Design review of the part built by this model. Coordinates are the model's own, in mm. A direction names the side the tool comes from. Coordinates: 2 decimals unless noted, no trailing zeros. Loops run counter-clockwise (first coordinate to the right, second up) from the corner with the lowest first, then second, coordinate; pieces in that order, holes last. Notation, with made-up numbers: M 43.25,33.25 L 91.25,33.25 A31 ccw 91.25,64.25 Z; hole C 66,45.25 d2. An arc over 180 degrees is marked long. One line per item, written item: value.
```python
from build123d import *

# Parameters (mm, degrees)
SKETCH1_R           = 1
BOSS_EXTRUDE1_DEPTH = 3
SKETCH2_R           = 5
CUT_EXTRUDE1_DEPTH  = 10
SKETCH4_W           = 3
SKETCH4_H           = 20
BOSS_EXTRUDE3_DEPTH = 3


with BuildPart() as part:
    # Sketch1 → Boss-Extrude1 (new body)
    with BuildSketch(Plane.XY):
        with BuildLine():
            Line((-16.174411119, 11.763860972), (32, 78))
            Line((32, 78), (32, 48))
            Line((32, 48), (19.455095298, -4.636730199))
            ThreePointArc((19.455095298, -4.636730199), (-8.362748941, -18.167675419), (-16.174411119, 11.763860972))
        make_face()
        with Locations((0, 16.5)):
            Circle(SKETCH1_R, mode=Mode.SUBTRACT)
        with Locations((-16.5, 0)):
            Circle(SKETCH1_R, mode=Mode.SUBTRACT)
        with Locations((0, -16.5)):
            Circle(SKETCH1_R, mode=Mode.SUBTRACT)
        with Locations((16.5, 0)):
            Circle(SKETCH1_R, mode=Mode.SUBTRACT)
    extrude(amount=-BOSS_EXTRUDE1_DEPTH)

    # Sketch2 → Cut-Extrude1 (cut)
    with BuildSketch(Plane.XY):
        Circle(SKETCH2_R)
    extrude(amount=-CUT_EXTRUDE1_DEPTH, mode=Mode.SUBTRACT)

    # Sketch4 → Boss-Extrude3 (add)
    with BuildSketch(Plane(origin=(32, 0, 0), x_dir=(0, 0, -1), z_dir=(1, 0, 0))):
        with Locations((1.5, 63)):
            Rectangle(SKETCH4_W, SKETCH4_H)
    extrude(amount=BOSS_EXTRUDE3_DEPTH)


solid = part.part
```
(1) To check wall thickness, follow line 1 along Y through (x, z) = (0, -1.2); line 2 along Y through (x, z) = (16.5, -1.05); line 3 along Y through (x, z) = (3.5, -1.1). State the ranges of each line that lie inside material, in increasing order. Write a range as [from, to].
Reply:
line 1: y = [-20, -17.5], [-15.5, -5], [5, 15.5], [17.5, 34]
line 2: y = [-11.3, -1], [1, 56.69]
line 3: y = [-19.69, -3.57], [3.57, 38.81]
(2) We need section A-A on y = -16.5. State the section outline as (x, z) points, then the cut area to 3 significant figures.
Reply:
outline: M -11.3,-3 L -1,-3 L -1,0 L -11.3,0 Z; M 1,-3 L 11.3,-3 L 11.3,0 L 1,0 Z
area: 61.8 mm2
(3) Insertion check: pin 1 (1.5 mm diameter, centred on x = 34, z = -1.5, fed in from +Y); pin 2 (1 mm diameter, centred on x = 12, z = -0.5, fed in from +Y); pin 3 (1.5 mm diameter, centred on x = 34, z = -1, fed in from -Y). Each pin has a flat end and moves straight along its axis. Give the tip position at first contact, or say it passes through.
Reply:
pin 1: stops at y = 73
pin 2: stops at y = 51.19
pin 3: stops at y = 53
(4) We need section C-C on x = 0. State the section outline as (y, z) points.
Reply:
outline: M -20,-3 L -17.5,-3 L -17.5,0 L -20,0 Z; M -15.5,-3 L -5,-3 L -5,0 L -15.5,0 Z; M 5,-3 L 15.5,-3 L 15.5,0 L 5,0 Z; M 17.5,-3 L 34,-3 L 34,0 L 17.5,0 Z
(5) Mouldability with a two-part tool opening along Y and no side actions: class faces 4 (the flat face through (8, 19, 0)), 5 (the flat face through (33, 73, -1)), 6 (the cylindrical face through (17.424, -0.383, -1.479)) as released by +Y, released by -Y, zero draft, split by the parting line, or undercut.
Reply:
face 4: zero draft
face 5: released by +Y
face 6: undercut
(6) We need section D-D on y = 0. State the section outline as (x, z) points, then the cut area to 3 significant figures.
Reply:
outline: M -20,-3 L -17.5,-3 L -17.5,0 L -20,0 Z; M -15.5,-3 L -5,-3 L -5,0 L -15.5,0 Z; M 5,-3 L 15.5,-3 L 15.5,0 L 5,0 Z; M 17.5,-3 L 20.56,-3 L 20.56,0 L 17.5,0 Z
area: 79.7 mm2
(7) Tool access review of faces 1 (the flat face through (32, 76, -1)), 2 (the flat face through (8, 19, -3)), 3 (the flat face through (33, 53, -1)): name each direction out of +Z, -Z, +X, -X, +Y, -Y from which nothing blocks a thin tool from reaching the whole face with its end or side.
Reply:
face 1: +Z, -Z, +X, +Y
face 2: -Z, +X, -X, +Y, -Y
face 3: +Z, -Z, +X, -Y
(8) We need section B-B on z = -0.9. State the section outline as (x, y) points, then the cut area to 3 significant figures.
Reply:
outline: M -16.17,11.76 A20 ccw long 19.46,-4.64 L 32,48 L 32,53 L 35,53 L 35,73 L 32,73 L 32,78 Z; hole C -16.5,0 d2; hole C 0,0 d10; hole C 0,-16.5 d2; hole C 0,16.5 d2; hole C 16.5,0 d2
area: 2,520 mm2
